from build123d import *

# Parameters (mm, degrees)
SKETCH1_W           = 79
SKETCH1_H           = 53
BOSS_EXTRUDE1_DEPTH = 2
SKETCH2_W           = 79
SKETCH2_H           = 53
SKETCH2_W_2         = 75
SKETCH2_H_2         = 49
BOSS_EXTRUDE2_DEPTH = 14
SKETCH3_W           = 79
SKETCH3_H           = 53
SKETCH3_W_2         = 77.4
SKETCH3_H_2         = 51.4
BOSS_EXTRUDE3_DEPTH = 2
SKETCH5_W           = 15
SKETCH5_H           = 16.5
CUT_EXTRUDE2_DEPTH  = 54
SKETCH6_W           = 15
SKETCH6_H           = 16.5
BOSS_EXTRUDE4_DEPTH = 2
SKETCH7_W           = 54
SKETCH7_H           = 15
BOSS_EXTRUDE6_DEPTH = 1
SKETCH8_W           = 15
SKETCH8_H           = 15.5
BOSS_EXTRUDE8_DEPTH = 2
FILLET1_R           = 1


with BuildPart() as part:
    # Sketch1 → Boss-Extrude1 (new body)
    with BuildSketch(Plane.XY):
        with Locations((39.5, 26.5)):
            Rectangle(SKETCH1_W, SKETCH1_H)
    extrude(amount=BOSS_EXTRUDE1_DEPTH)

    # Sketch2 → Boss-Extrude2 (add)
    with BuildSketch(Plane.XY.offset(2)):
        with Locations((39.5, 26.5)):
            Rectangle(SKETCH2_W, SKETCH2_H)
        with Locations((39.5, 26.5)):
            Rectangle(SKETCH2_W_2, SKETCH2_H_2, mode=Mode.SUBTRACT)
    extrude(amount=BOSS_EXTRUDE2_DEPTH)

    # Sketch3 → Boss-Extrude3 (add)
    with BuildSketch(Plane.XY.offset(16)):
        with Locations((39.5, 26.5)):
            Rectangle(SKETCH3_W, SKETCH3_H)
        with Locations((39.5, 26.5)):
            Rectangle(SKETCH3_W_2, SKETCH3_H_2, mode=Mode.SUBTRACT)
    extrude(amount=BOSS_EXTRUDE3_DEPTH)

    # Sketch5 → Cut-Extrude2 (cut)
    with BuildSketch(Plane.ZY.offset(-5)):
        with Locations((7.5, 8.25)):
            Rectangle(SKETCH5_W, SKETCH5_H)
    extrude(amount=-CUT_EXTRUDE2_DEPTH, mode=Mode.SUBTRACT)

    # Sketch6 → Boss-Extrude4 (add)
    with BuildSketch(Plane.ZY.offset(-59)):
        with Locations((7.5, 8.25)):
            Rectangle(SKETCH6_W, SKETCH6_H)
    extrude(amount=-BOSS_EXTRUDE4_DEPTH)

    # Sketch7 → Boss-Extrude6 (add)
    with BuildSketch(Plane.XZ.offset(-16.5)):
        with Locations((32, 7.5)):
            Rectangle(SKETCH7_W, SKETCH7_H)
    extrude(amount=BOSS_EXTRUDE6_DEPTH)

    # Sketch8 → Boss-Extrude8 (add)
    with BuildSketch(Plane(origin=(5, 0, 0), x_dir=(0, 0, -1), z_dir=(1, 0, 0))):
        with Locations((-7.5, 7.75)):
            Rectangle(SKETCH8_W, SKETCH8_H)
    extrude(amount=BOSS_EXTRUDE8_DEPTH)

    # Fillet1
    fillet1_edges = [part.edges().sort_by_distance(p)[0] for p in [
        (59, 7.75, 0),
        (5, 16.5, 8.5),
        (59, 15.5, 7.5),
        (33, 15.5, 0),
        (7, 7.75, 0),
        (7, 15.5, 7.5),
        (7, 0, 7.5),
        (77, 26.5, 2),
        (39.5, 51, 2),
        (2, 26.5, 2),
        (3.5, 2, 2),
        (77, 51, 9),
        (2, 51, 9),
        (2, 2, 9),
        (77, 2, 9),
        (78.2, 52.2, 17),
        (0.8, 52.2, 17),
        (0.8, 0.8, 17),
        (78.2, 0.8, 17),
        (39.5, 53, 0),
        (79, 26.5, 0),
        (3.5, 0, 0),
        (0, 26.5, 0),
        (69, 0, 0),
        (33, 16.5, 2),
        (5, 9.25, 2),
        (59, 0, 7.5),
        (5, 2, 8.5),
        (0, 53, 9),
        (79, 53, 9),
        (79, 0, 9),
        (0, 0, 9),
        (69, 2, 2),
        (61, 9.25, 2),
        (61, 16.5, 8.5),
        (61, 2, 8.5),
    ]]
    fillet(fillet1_edges, radius=FILLET1_R)


solid = part.part
Work out the finished part from the listing and answer in its coordinate system (mm). A direction names the side the tool comes from. Give positions to 0.01 mm unless a question says otherwise; leave off trailing zeros. Loops run counter-clockwise (first coordinate to the right, second up) from the corner with the lowest first, then second, coordinate; pieces in that order, holes last. Notation, with made-up numbers: (6.25, -25.75) -> (33.25, -25.75) arc R23 cw to (33.25, 9.25) -> close; hole circle Ø6 at (-19, 21.25). An arc over 180 degrees is marked (long way). Use a Markdown table: item, result. Add a question column.
1. Section B-B on x = 13 is taken. Determine the outline of the cut face in (y, z).
2. Find the intervals of material crossed by probe 1 along X at (y, z) = (5, 11.25); probe 2 along X at (y, z) = (37, 8.5); probe 3 along Y at (x, z) = (50.5, 16.75), in increasing order.
3. Section D-D on y = 49 is taken. Determine the outline of the cut face in (x, z).
4. Flat-ended cylindrical pins translate along their axes: pin 1 Ø4 at (x, z) = (35, 6.5) entering from -Y; pin 2 Ø5 at (x, y) = (15.5, 21.5) entering from +Z. Find the tip coordinate at first contact, or state that the pin passes through.
5. Section A-A on y = 9.5 is taken. Determine the outline of the cut face in (x, z).
6. For faces 5 (the flat face through (47.5, 0, 15.3)), 6 (the flat face through (33, 1, 15)), 7 (the flat face through (0.8, 26, 17)), determine the directions among +Z, -Z, +X, -X, +Y, -Y from which every point of the face is accessible in a straight line to the end or side of a thin tool.
7. Determine the mould class of faces 1 (the flat face through (39, 53, 9)), 2 (the flat face through (39, 32, 0)), 3 (the flat face through (33, 15.5, 8)), 4 (the flat face through (77, 26, 9)) for opening direction Y: released by +Y, released by -Y, zero draft, split by the parting line, or undercut.
Results below:
| question | item | result |
|---|---|---|
| 1 | outline | (0, 15) -> (2, 15) -> (2, 16) -> (0.8, 16) -> (0.8, 18) -> (0, 18) -> close; (15.5, 1) arc R1 ccw to (16.5, 0) -> (52, 0) arc R1 ccw to (53, 1) -> (53, 18) -> (52.2, 18) -> (52.2, 16) -> (51, 16) -> (51, 3) arc R1 cw to (50, 2) -> (17.5, 2) arc R1 cw to (16.5, 3) -> (16.5, 15) -> (15.5, 15) -> close |
| 2 | probe 1 | x = 0 to 2, 5 to 7, 59 to 61, 77 to 79 |
| 2 | probe 2 | x = 0 to 2, 77 to 79 |
| 2 | probe 3 | y = 0 to 0.8, 52.2 to 53 |
| 3 | outline | (0, 1) arc R1 ccw to (1, 0) -> (78, 0) arc R1 ccw to (79, 1) -> (79, 18) -> (78.2, 18) -> (78.2, 16) -> (77, 16) -> (77, 3) arc R1 cw to (76, 2) -> (3, 2) arc R1 cw to (2, 3) -> (2, 16) -> (0.8, 16) -> (0.8, 18) -> (0, 18) -> close |
| 4 | pin 1 | stops at y = 15.5 |
| 4 | pin 2 | stops at z = 2 |
| 5 | outline | (0, 1) arc R1 ccw to (1, 0) -> (6, 0) arc R1 ccw to (7, 1) -> (7, 15) -> (5, 15) -> (5, 3) arc R1 cw to (4, 2) -> (3, 2) arc R1 cw to (2, 3) -> (2, 16) -> (0.8, 16) -> (0.8, 18) -> (0, 18) -> close; (59, 1) arc R1 ccw to (60, 0) -> (78, 0) arc R1 ccw to (79, 1) -> (79, 18) -> (78.2, 18) -> (78.2, 16) -> (77, 16) -> (77, 3) arc R1 cw to (76, 2) -> (62, 2) arc R1 cw to (61, 3) -> (61, 15) -> (59, 15) -> close |
| 6 | face 5 | +Z, -Z, +X, -X, -Y |
| 6 | face 6 | -Z, -Y |
| 6 | face 7 | +Z |
| 7 | face 1 | released by +Y |
| 7 | face 2 | zero draft |
| 7 | face 3 | released by -Y |
| 7 | face 4 | undercut |
